Autodesk Inventor part; units mm, degrees
ref_plane "YZ Plane" through (0, 0, 0) normal (1, 0, 0) x (0, 1, 0)
ref_plane "XZ Plane" through (0, 0, 0) normal (0, 1, 0) x (-1, 0, 0)
ref_plane "XY Plane" through (0, 0, 0) normal (0, 0, 1) x (1, 0, 0)
sketch "Sketch1" plane through (0, 0, 0) normal (0, 1, 0) x (-1, 0, 0)
  line L0 (0, 0) -> (-5, 0)
  line L1 (-5, 0) -> (-5, 3.5)
  line L2 (-0.5, 3.5) -> (0, 3.5)
  line L3 (0, 3.5) -> (0, 0)
  line L4 (-5, 0) -> (-4.5, 0)
  line L5 (-4.5, 7.5) -> (-4.5, 11)
  line L6 (-4.5, 11) -> (-5, 11)
  line L7 (-5, 11) -> (-5, 0)
  arc A0 (-4.5, 7.5) -> (-0.5, 3.5) centre (-0.5, 7.5) ccw
  dimension "d0" = 5
  dimension "d1" = 3.5
  dimension "d2" = 0.5
  dimension "d3" = 11
  dimension "d4" = 4
extrude "Extrusion1" add sketch "Sketch1" along normal blind 3.5
sketch "Sketch2" plane through (0, 3.5, 0) normal (0, 1, 0) x (1, 0, 0)
  line L0 (0, -3.5) -> (0.5, -3.5)
  line L1 (5, -11) -> (5, 0)
  line L2 (0, -3.5) -> (5, -3.5)
  line L3 (5, -3.5) -> (5, 0)
  line L4 (5, 0) -> (0, 0)
  line L5 (0, 0) -> (0, -3.5)
  circle A0 centre (1.551, -1.75) radius 0.75
  dimension "d7" = 1.5
extrude "Extrusion2" cut sketch "Sketch2" against normal blind 3.5 contours A0
sketch "Sketch3" plane through (0, 0, 0) normal (0, -1, 0) x (1, 0, 0)
  line L0 (5, 11) -> (5, 0)
  arc A0 (0.5, 3.5) -> (4.5, 7.5) centre (0.5, 7.5) ccw
  line L1 (5, 11) -> (4.5, 11)
  line L2 (4.5, 11) -> (4.5, 7.5)
  line L3 (4.5, 7.5) -> (5, 7.5)
  line L4 (5, 7.5) -> (5, 11)
  line L5 (5, 0) -> (0, 0)
  line L6 (5, 7.5) -> (4.5, 7.5)
  line L7 (4.5, 7.5) -> (4.5, 0)
  line L8 (4.5, 0) -> (5, 0)
  line L9 (5, 0) -> (5, 7.5)
extrude "Extrusion3" add sketch "Sketch3" along normal blind 4.8
sketch "Sketch4" plane through (0, 3.5, 0) normal (0, 1, 0) x (1, 0, 0)
  line L0 (5, -11) -> (4.5, -11)
  circle A0 centre (4.75, -11) radius 0.4
  point P0 (0, 0)
  dimension "d12" = 0.8
extrude "Extrusion4" add sketch "Sketch4" along normal blind 0.3 and the other way blind 8.3
sketch "Sketch5" plane through (0, -4.8, 0) normal (0, -1, 0) x (1, 0, 0)
  circle A0 centre (4.75, 11) radius 0.4
  line L0 (4.6264, 10.6196) -> (0.9709, 20.663)
  line L1 (4.6264, 10.6196) -> (15.3144, 10.6196) construction
  line L2 (0.9709, 20.663) -> (1.4407, 20.834)
  line L3 (1.4407, 20.834) -> (5.0551, 11.2587)
  point P0 (0, 0)
  point P1 (4.4108, 11.212)
  dimension "d17" = 10.688
  dimension "d18" = 110
  dimension "d19" = 0.5
extrude "Extrusion5" add sketch "Sketch5" against normal blind 8.3 contours A0 L0 L2 L3
chamfer "Chamfer1" distance 0.5 angle 45 1 edges at (1.4407, -0.65, 20.834)
sketch "Sketch6" plane through (5, -4.8, 0) normal (1, 0, 0) x (0, 0, -1)
  point P0 (0, 4.8)
properties part number "McCrea_finger_Walle"
Verification items for the finished model (mm, model axes). A direction names the side the tool comes from. Give positions to 0.01 mm unless a question says otherwise; leave off trailing zeros. Loops run counter-clockwise (first coordinate to the right, second up) from the corner with the lowest first, then second, coordinate; pieces in that order, holes last. Notation, with made-up numbers: M 78,-33.75 L 99,-33.75 A19 cw 99,-24.75 Z; hole C 76.25,21 d3. An arc over 180 degrees is marked long. Return JSON: item names as keys, results as strings.
1) Section check A-A, the plane z = 1.75. Enter the section's corners in (x, y), and give its area (4 significant figures).
Findings:
{"outline": "M 0,0 L 0.8,0 L 0.8,3.5 L 0,3.5 Z; M 2.3,0 L 4.5,0 L 4.5,-4.8 L 5,-4.8 L 5,3.5 L 2.3,3.5 Z", "area": "14.65 mm2"}
2) Tool access check on faces 1 (the cylindrical face through (3.297, 1.726, 4.641)), 2 (the flat face through (4.5, -2, 6)), 3 (the flat face through (3, 0, 2)), 4 (the flat face through (5, -1, 5)). Record the directions out of +Z, -Z, +X, -X, +Y, -Y that give a thin tool (end or side, any length) a straight path to the whole face; none if there is none.
Findings:
{"face 1": "-X, +Y, -Y", "face 2": "-X, -Y", "face 3": "-Z, -X, -Y", "face 4": "-Z, +X, +Y, -Y"}
3) Section check B-B, the plane x = 1.85. Enter the section's corners in (y, z).
Findings:
{"outline": "M -4.8,18.25 L 3.5,18.25 L 3.5,19.75 L -4.8,19.75 Z; M 0,0 L 3.5,0 L 3.5,1.06 L 0,1.06 Z; M 0,2.44 L 3.5,2.44 L 3.5,3.73 L 0,3.73 Z"}
4) Mould release check, pull along Y, two halves, no side actions. Record for faces 5 (the flat face through (5, -4.8, 11)), 6 (the flat face through (2, 1, 0)), 7 (the flat face through (5, 3.8, 11)): released by +Y, released by -Y, zero draft, split by the parting line, or undercut.
Findings:
{"face 5": "released by -Y", "face 6": "zero draft", "face 7": "released by +Y"}
5) Gauge pin test, flat ends, axial feed: P1, Ø2, axis at x = 1, z = 6.5, coming from the +Y side; P2, Ø4, axis at y = 1.5, z = 4, coming from the +X side; P3, Ø1.7, axis at x = 1.551, z = 1.75, coming from the +Y side. Record the tip position at first contact, or that the pin passes through.
Findings:
{"P1": "passes through", "P2": "stops at x = 5", "P3": "stops at y = 3.5"}
6) Material ranges on L1, parallel to X at y = 2.4, z = 1.75; L2, parallel to Y at x = 4.65, z = 8.5; L3, parallel to Y at x = 2.9, z = 1.5, recorded low to high. Write a range as [from, to].
Findings:
{"L1": "x = [0, 0.8], [2.3, 5]", "L2": "y = [-4.8, 3.5]", "L3": "y = [0, 3.5]"}
7) Section check C-C, the plane x = 2.7. Enter the section's corners in (y, z).
Findings:
{"outline": "M -4.8,15.91 L 3.5,15.91 L 3.5,17.5 L -4.8,17.5 Z; M 0,0 L 3.5,0 L 3.5,4.16 L 0,4.16 Z"}
